Could you check a few things on this drawing? It's one solid part, dimensions in mm from its lowest x, y, z. A direction names the side the tool comes from. Coordinates: 2 decimals unless noted, no trailing zeros. Order: outer loops, then holes, each group sorted by start corner. A loop starts at its lowest first (then second) coordinate and runs counter-clockwise, first axis right, second up. Notation, with made-up numbers: (-22, 77) - (3, 77) arc R32 ccw to (3, 116) - close; hole circle Ø3 at (1, 25). An arc over 180 degrees is marked (long way). Return JSON: item names as keys, results as strings. Group by question number.
1) For pin 1 Ø1.5 at (y, z) = (2.5, 11.5) entering from +X, with a flat end and sliding along its axis, tell me the tip position at first contact or that it passes through.
2) If we mould it in two halves opening along Z, with no side actions, what happens to the marked faces 1, 2, 3 and 4? For each: pulls with the +Z half, pulls with the -Z half, needs draft (parallel to the pull), parting line crosses it, or undercut.
3) Imagine slicing it at A-A (z = 10.25). Write out the boundary of the cut face in (x, y).
4) Imagine slicing it at D-D (y = 0.5). Write out the boundary of the cut face in (x, z) (1 decimal).
5) If I drill on line 1 along Y through (x, z) = (17.75, 17.5); line 2 along X through (y, z) = (1.1, 13); line 3 along X through (y, z) = (5, 11) (1 decimal), over which ranges is the centre line in solid material (lowest first)?
6) Imagine slicing it at C-C (x = 3.25). Write out the boundary of the cut face in (y, z), and give its area (3 significant figures).
7) Which directions (+Z, -Z, +X, -X, +Y, -Y) give clear straight access to the entire face, cutting with the end or side of a thin tool? Please do the marked faces 5 and 6.
8) Imagine slicing it at B-B (x = 15.5). Write out the boundary of the cut face in (y, z), and give its area (3 significant figures).
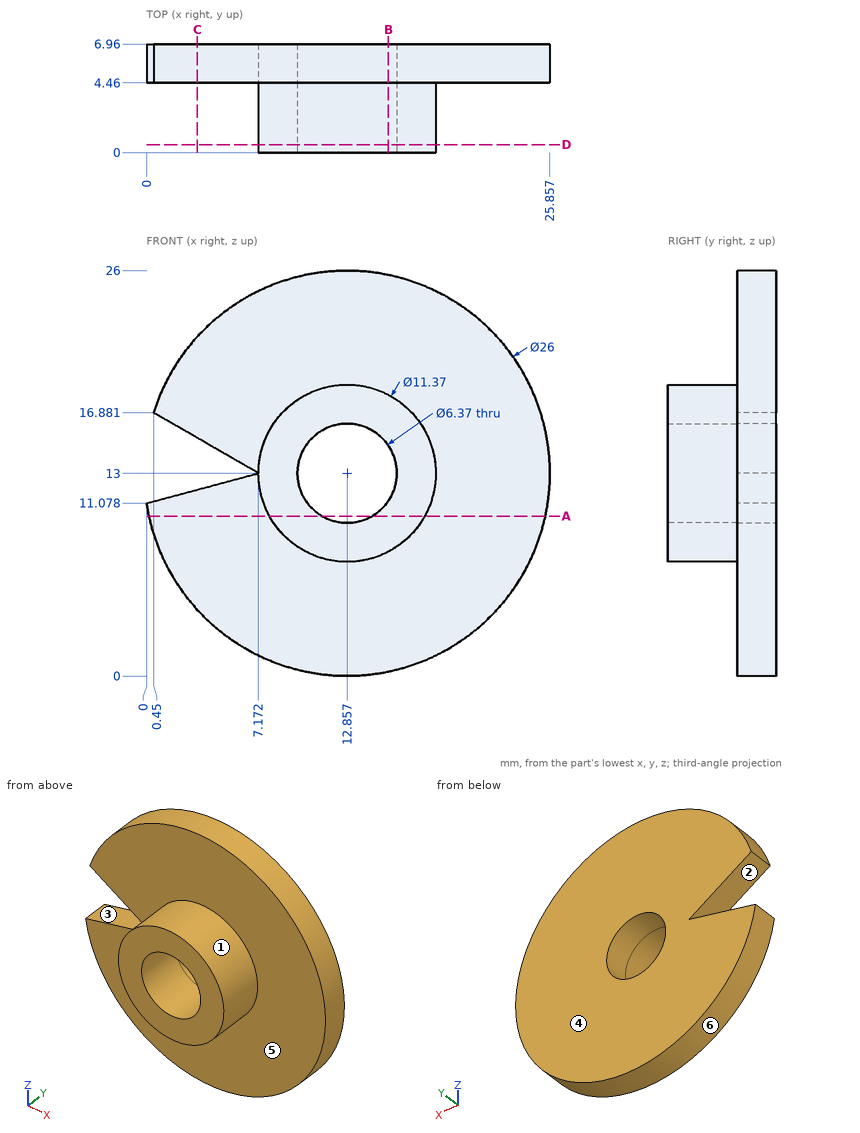
Calculated:
{
 "1": {"pin 1": "x = 18.49"},
 "2": {"face 1": "parting line crosses it", "face 2": "undercut", "face 3": "undercut", "face 4": "needs draft"},
 "3": {"outline": "(0.15, 4.46) - (7.88, 4.46) - (7.88, 0) - (11.25, 0) - (11.25, 6.96) - (0.15, 6.96) - close; (14.46, 0) - (17.83, 0) - (17.83, 4.46) - (25.56, 4.46) - (25.56, 6.96) - (14.46, 6.96) - close"},
 "4": {"outline": "circle Ø11.4 at (12.9, 13); hole circle Ø6.4 at (12.9, 13)"},
 "5": {"line 1": "4.46 to 6.96", "line 2": "7.17 to 9.67, 16.04 to 18.54", "line 3": "0 to 10.4, 15.3 to 25.7"},
 "6": {"outline": "(4.46, 4.24) - (6.96, 4.24) - (6.96, 11.95) - (4.46, 11.95) - close; (4.46, 15.26) - (6.96, 15.26) - (6.96, 21.76) - (4.46, 21.76) - close", "area": "35.5 mm2"},
 "7": {"face 5": "-Y", "face 6": "+Y, -Y"},
 "8": {"outline": "(0, 7.97) - (4.46, 7.97) - (4.46, 0.27) - (6.96, 0.27) - (6.96, 11.22) - (0, 11.22) - close; (0, 14.78) - (6.96, 14.78) - (6.96, 25.73) - (4.46, 25.73) - (4.46, 18.03) - (0, 18.03) - close", "area": "83.8 mm2"}
}
